Check sheet for the modelled part. Datum: model origin and axes. Units: mm. A direction names the side the tool comes from. Give positions to 0.01 mm unless a question says otherwise; leave off trailing zeros. Order: outer loops, then holes, each group sorted by start corner. A loop starts at its lowest first (then second) coordinate and runs counter-clockwise, first axis right, second up. Notation, with made-up numbers: (65.5, 30.5) -> (82.5, 30.5) arc R19 ccw to (82.5, 63.5) -> close; hole circle Ø9 at (23, 1). An arc over 180 degrees is marked (long way). Write each question's results on one line, items separated by ' | '.
from build123d import *

# Parameters (mm, degrees)
SKETCH1_W               = 50.8
SKETCH1_H               = 50.8
BOSS_EXTRUDE1_DEPTH     = 3.175
SKETCH2_W               = 12.7
SKETCH2_H               = 13.208
SKETCH2_R               = 1.5875
BOSS_EXTRUDE2_DEPTH     = 3.175
LPATTERN1_COUNT         = 2
LPATTERN1_PITCH         = 25.4
MIRROR1_COPY_1_SKETCH_W = 12.7
MIRROR1_COPY_1_SKETCH_H = 13.208
MIRROR1_COPY_1_SKETCH_R = 1.5875
MIRROR1_COPY_1_DEPTH    = 3.175


with BuildPart() as part:
    # Sketch1 → Boss-Extrude1 (new body)
    with BuildSketch(Plane(origin=(0, 0, 0), x_dir=(1, 0, 0), z_dir=(0, 1, 0))):
        with Locations((25.4, 25.4)):
            Rectangle(SKETCH1_W, SKETCH1_H)
    extrude(amount=BOSS_EXTRUDE1_DEPTH)

    # Sketch2 → Boss-Extrude2 (add)
    with BuildSketch(Plane(origin=(0, 3.175, 0), x_dir=(1, 0, 0), z_dir=(0, 1, 0))):
        with Locations((57.15, 44.196)):
            Rectangle(SKETCH2_W, SKETCH2_H)
        with Locations((57.15, 43.942)):
            Circle(SKETCH2_R, mode=Mode.SUBTRACT)
    boss_extrude2 = extrude(amount=-BOSS_EXTRUDE2_DEPTH)

    # LPattern1: Boss-Extrude2 ×2
    with Locations(*[(0, 0, i * LPATTERN1_PITCH) for i in range(1, LPATTERN1_COUNT)]):
        add(boss_extrude2)

    # Mirror1: Boss-Extrude2 across plane
    add(boss_extrude2.mirror(Plane.ZY.offset(-25.4)))

    # Mirror1 copy 1 sketch → Mirror1 copy 1 (add)
    with BuildSketch(Plane(origin=(50.8, 3.175, 25.4), x_dir=(-1, 0, 0), z_dir=(0, 1, 0))):
        with Locations((57.15, -44.196)):
            Rectangle(MIRROR1_COPY_1_SKETCH_W, MIRROR1_COPY_1_SKETCH_H)
        with Locations((57.15, -43.942)):
            Circle(MIRROR1_COPY_1_SKETCH_R, mode=Mode.SUBTRACT)
    extrude(amount=-MIRROR1_COPY_1_DEPTH)


solid = part.part
1. Section check A-A on x = 57.15. Record the cut outline in (y, z) (1 decimal), then the cut area to 3 significant figures.
Verdict:
outline: (0, -50.8) -> (3.2, -50.8) -> (3.2, -45.5) -> (0, -45.5) -> close; (0, -42.4) -> (3.2, -42.4) -> (3.2, -37.6) -> (0, -37.6) -> close; (0, -25.4) -> (3.2, -25.4) -> (3.2, -20.1) -> (0, -20.1) -> close; (0, -17) -> (3.2, -17) -> (3.2, -12.2) -> (0, -12.2) -> close | area: 63.7 mm^2
2. Section check B-B on z = -30. Record the cut outline in (x, y) (3 decimals), then the cut area to 3 significant figures.
Verdict:
outline: (0, 0) -> (50.8, 0) -> (50.8, 3.175) -> (0, 3.175) -> close | area: 161 mm^2
3. Section check C-C on y = 2.45. Give the number of separate pieces and of enclosed holes in the cut face, then the cut area to 3 significant figures.
Verdict:
separate pieces: 1 | enclosed holes: 4 | area: 3,220 mm^2
4. Access from +Z, -Z, +X, -X, +Y, -Y to the whole of each face (thin tool, end or side, straight path). Record for faces 4 (the flat face through (57, 2, -12.192)), 5 (the flat face through (57, 2, -37.592)), 6 (the flat face through (-12.7, 2, -44)), 7 (the flat face through (-6, 2, -12.192)), 8 (the flat face through (-6, 2, -37.592)).
Verdict:
face 4: +Z, +X, +Y, -Y | face 5: +X, +Y, -Y | face 6: +Z, -Z, -X, +Y, -Y | face 7: +Z, -X, +Y, -Y | face 8: -X, +Y, -Y
5. Material ranges on probe 1 along Z at (x, y) = (57.15, 0.9); probe 2 along X at (y, z) = (1.55, -28.5); probe 3 along X at (y, z) = (0.2, -42.5), recorded low to high. Write a range as from..to.
Verdict:
probe 1: z = -50.8..-45.53, -42.35..-37.59, -25.4..-20.13, -16.95..-12.19 | probe 2: x = 0..50.8 | probe 3: x = -12.7..-7.01, -5.69..56.49, 57.81..63.5
6. Gauge pin test, flat ends, axial feed: pin 1 Ø1.6 at (y, z) = (1, -5) entering from -X; pin 2 Ø1.6 at (y, z) = (1, -4.5) entering from +X; pin 3 Ø2 at (x, z) = (5, -43.5) entering from -Y. Record the tip position at first contact, or that the pin passes through.
Verdict:
pin 1: stops at x = 0 | pin 2: stops at x = 50.8 | pin 3: stops at y = 0
7. Mould release check, pull along Z, two halves, no side actions. Record for faces 1 (the flat face through (26, 3.175, -26)), 2 (the flat face through (25, 2, 0)), 3 (the flat face through (-6, 2, -25.4)): +Z half, -Z half, draft (parallel to the pull), parting line (faces both ways), or undercut.
Verdict:
face 1: draft | face 2: +Z half | face 3: undercut
